```python
from build123d import *

# Parameters (mm, degrees)
F2_R    = 1
F3_SIZE = 1


with BuildPart() as f1:
    # F0 (on Front) → F1 (revolve)
    with BuildSketch(Plane.XZ):
        Polygon((4, 16.67762), (0.6, 16.67762), (0.6, -11.32238), (7.5, -11.32238), (8, 3.67762), (12, 3.67762), (12, 6.67762), (4, 6.67762), align=None)
    revolve(axis=Axis((0, 0, 0.295774), (0, 0, -1)))

    # F2
    f2_edges = [f1.edges().sort_by_distance(p)[0] for p in [
        (-8, 0, 3.67762),
        (-12, 0, 3.67762),
        (-12, 0, 6.67762),
        (-4, 0, 16.67762),
        (-4, 0, 6.67762),
    ]]
    fillet(f2_edges, radius=F2_R)

    # F3
    f3_edges = [f1.edges().sort_by_distance(p)[0] for p in [
        (-7.5, 0, -11.32238),
    ]]
    chamfer(f3_edges, length=F3_SIZE)


solid = f1.part
```
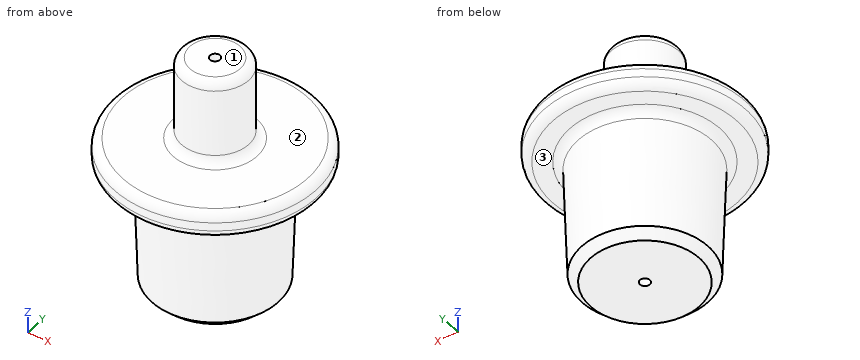
Source: CAD feature listing. Evaluate the final solid. Frame: model axes, mm. Face numbers are marked on the shaded views. A direction names the side the tool comes from. Give positions to 0.01 mm unless a question says otherwise; leave off trailing zeros. Write each loop counter-clockwise with the first axis right and the second up, starting at its lowest first coordinate (ties: lowest second). Pieces come first, ordered by that corner, then holes.
1. Material intervals for line 1 along X through (y, z) = (0, 7.75); line 2 along X through (y, z) = (0, 1.75), sorted ascending.
2. Section query D-D (z = -9.25). Return the cut outline in (x, y), then the cut area to 3 significant figures.
3. Access query for the marked faces 1, 2 and 3. Directions: +Z, -Z, +X, -X, +Y, -Y. A direction counts if a zero-diameter tool reaches every point of the face in a straight line with its end or side. Return the directions, or none.
4. First-contact query: pin 1 (12 mm diameter, centred on x = 8.5, z = -8, fed in from -Y); pin 2 (4 mm diameter, centred on x = -5, z = 7.5, fed in from -Y); pin 3 (2 mm diameter, centred on x = -7, y = 8.5, fed in from +Z); pin 4 (5 mm diameter, centred on x = 1, z = 4.5, fed in from +Y). Flat tips, straight axial feed; report the tip coordinate or a pass-through.
5. Section query A-A (x = 0). Return the cut outline in (y, z).
6. Section query C-C (z = -5.75). Return the cut outline in (x, y), then the cut area to 3 significant figures.
Output values:
1. line 1: x = -4 to -0.6, 0.6 to 4
1. line 2: x = -7.94 to -0.6, 0.6 to 7.94
2. outline: circle Ø15.14 at (0, 0); hole circle Ø1.2 at (0, 0)
2. area: 179 mm2
3. face 1: +Z, +X, -X, +Y, -Y
3. face 2: +Z
3. face 3: -Z
4. pin 1: stops at y = -7.2
4. pin 2: stops at y = -11.37
4. pin 3: stops at z = 6.68
4. pin 4: stops at y = 12
5. outline: (-12, 4.68) arc R1 ccw to (-11, 3.68) - (-8.97, 3.68) arc R1 cw to (-7.97, 2.71) - (-7.53, -10.32) - (-6.5, -11.32) - (-0.6, -11.32) - (-0.6, 16.68) - (-3, 16.68) arc R1 ccw to (-4, 15.68) - (-4, 7.68) arc R1 cw to (-5, 6.68) - (-11, 6.68) arc R1 ccw to (-12, 5.68) - close; (0.6, -11.32) - (6.5, -11.32) - (7.53, -10.32) - (7.97, 2.71) arc R1 cw to (8.97, 3.68) - (11, 3.68) arc R1 ccw to (12, 4.68) - (12, 5.68) arc R1 ccw to (11, 6.68) - (5, 6.68) arc R1 cw to (4, 7.68) - (4, 15.68) arc R1 ccw to (3, 16.68) - (0.6, 16.68) - close
6. outline: circle Ø15.37 at (0, 0); hole circle Ø1.2 at (0, 0)
6. area: 184 mm2
